Work out the finished part from the listing and answer in its coordinate system (mm). A direction names the side the tool comes from. Round coordinates to 2 decimals unless told otherwise and drop trailing zeros. Order: outer loops, then holes, each group sorted by start corner. A loop starts at its lowest first (then second) coordinate and runs counter-clockwise, first axis right, second up. Notation, with made-up numbers: (55.25, 14) - (111.25, 14) arc R17 ccw to (111.25, 30) - close; hole circle Ø11 at (-9, 39). An arc over 180 degrees is marked (long way). Put each result on its own line as item: value.
```python
from build123d import *

# Parameters (mm, degrees)
F1_DEPTH      = 50
F1_DEPTH_BACK = 50


with BuildPart() as f1:
    # F0 (on Right) → F1 (new body, two sides)
    with BuildSketch(Plane.YZ) as f1_sk:
        Polygon((0, 20), (0, 0), (70, 0), (70, 90), (50, 90), (50, 20), align=None)
    extrude(amount=F1_DEPTH)
    extrude(f1_sk.sketch, amount=-F1_DEPTH_BACK)


solid = f1.part
```
1) For faces 1 (the flat face through (1, 50, 55)), 2 (the flat face through (1, 60, 90)), determine the directions among +Z, -Z, +X, -X, +Y, -Y from which every point of the face is accessible in a straight line to the end or side of a thin tool.
Findings below:
face 1: +Z, +X, -X, -Y
face 2: +Z, +X, -X, +Y, -Y
2) Straight lines are drawn through the part: L1, parallel to Z at x = -23.5, y = 24.5; L2, parallel to Y at x = -39, z = 34.5. For each, find the intervals that lie inside material, in ascending order. Write a range as from..to.
Findings below:
L1: z = 0..20
L2: y = 50..70
3) A cutting plane is placed at B-B on y = 12.5. Write down the section's boundary in (x, z).
Findings below:
outline: (-50, 0) - (50, 0) - (50, 20) - (-50, 20) - close
4) A cutting plane is placed at A-A on x = 40. Write down the section's boundary in (y, z).
Findings below:
outline: (0, 0) - (70, 0) - (70, 90) - (50, 90) - (50, 20) - (0, 20) - close
5) A cutting plane is placed at C-C on z = 34.5. Write down the section's boundary in (x, y).
Findings below:
outline: (-50, 50) - (50, 50) - (50, 70) - (-50, 70) - close
6) Given pin 1 Ø5 at (x, z) = (-38.5, 36) entering from -Y; pin 2 Ø8 at (x, y) = (-14.5, 40) entering from +Z, each flat-ended and moving along its own axis, determine where each tip first touches the part or whether it passes through.
Findings below:
pin 1: stops at y = 50
pin 2: stops at z = 20
